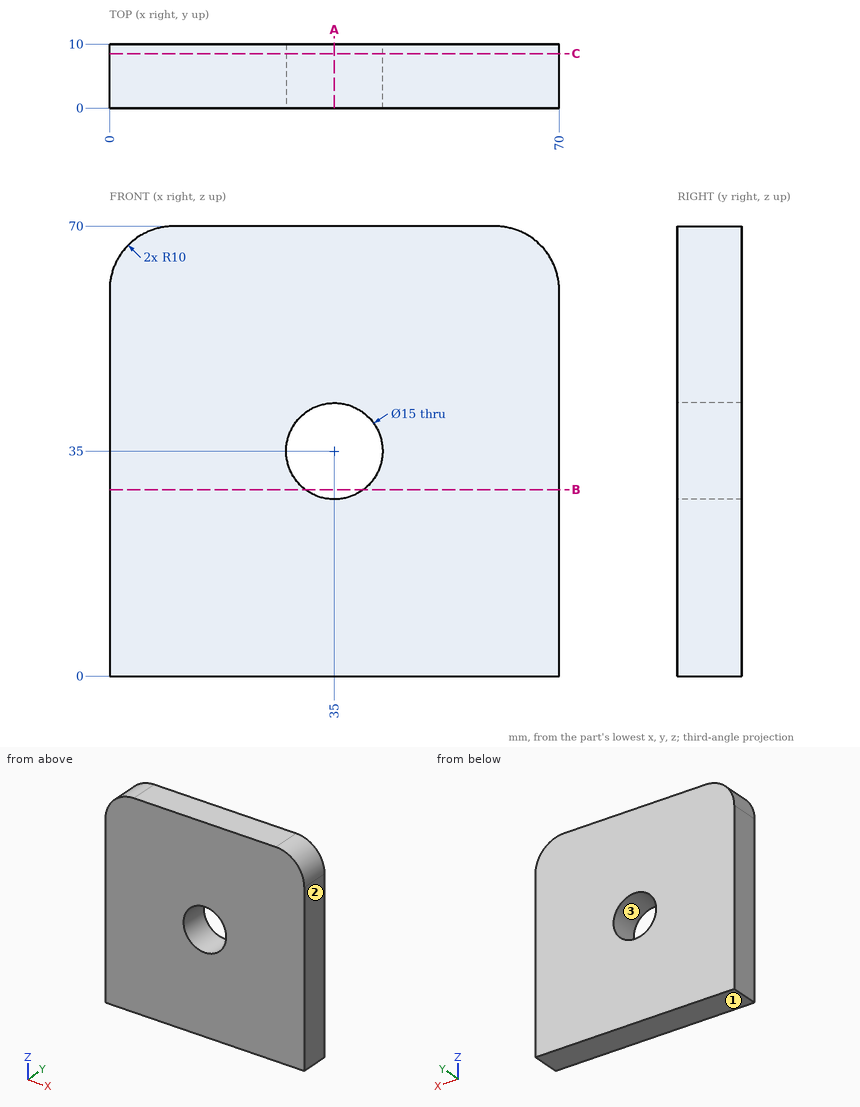
Input: dimensioned drawing with shaded views. Units: mm. Origin: part minimum x, y, z. Round coordinates to 2 decimals unless told otherwise and drop trailing zeros. Order: outer loops, then holes, each group sorted by start corner. A loop starts at its lowest first (then second) coordinate and runs counter-clockwise, first axis right, second up.
1. Mould query, pull axis Z, two halves, no side actions, for the marked faces 1, 2 and 3. Classes: released by +Z, released by -Z, zero draft, split by the parting line, or undercut.
The answers:
face 1: released by -Z
face 2: zero draft
face 3: undercut
2. Cut plane A-A, the plane x = 35. Output: boundary loops of the cut face in (y, z), then the cut area to 3 significant figures.
The answers:
outline: (0, 0) - (10, 0) - (10, 27.5) - (0, 27.5) - close; (0, 42.5) - (10, 42.5) - (10, 70) - (0, 70) - close
area: 550 mm2
3. Material intervals for line 1 (Z direction, x = 35, y = 7); line 2 (Z direction, x = 8, y = 4), sorted ascending.
The answers:
line 1: z = 0 to 27.5, 42.5 to 70
line 2: z = 0 to 69.8
4. Cut plane C-C, the plane y = 8.5. Output: boundary loops of the cut face in (x, z).
The answers:
outline: (0, 0) - (70, 0) - (70, 60) arc R10 ccw to (60, 70) - (10, 70) arc R10 ccw to (0, 60) - close; hole circle Ø15 at (35, 35)
5. Pin query (flat end, axial travel): P1, Ø5, axis at y = 7.5, z = 34, coming from the -X side. Return the tip coordinate at first contact, or that it passes through.
The answers:
P1: stops at x = 0
6. Cut plane B-B, the plane z = 29. Output: boundary loops of the cut face in (x, y), then the cut area to 3 significant figures.
The answers:
outline: (0, 0) - (30.5, 0) - (30.5, 10) - (0, 10) - close; (39.5, 0) - (70, 0) - (70, 10) - (39.5, 10) - close
area: 610 mm2
